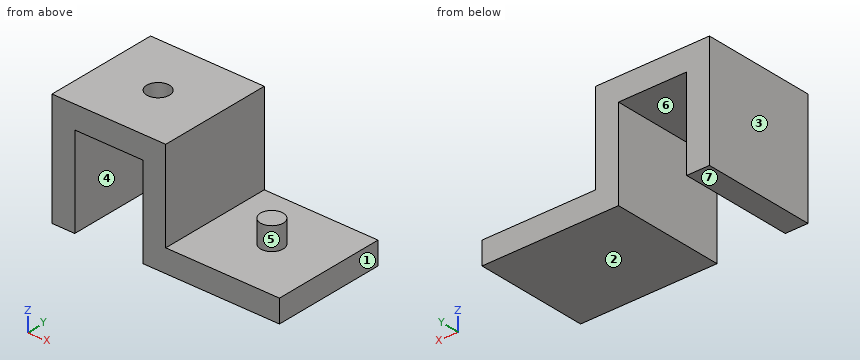
```python
from build123d import *

# Parameters (mm, degrees)
F1_DEPTH = 50
F2_W     = 30
F2_H     = 40
F3_DEPTH = 50.001
F4_R     = 5
F5_DEPTH = 50.001
F6_R     = 5
F7_DEPTH = 10


with BuildPart() as f1:
    # F0 (on Front) → F1 (new body)
    with BuildSketch(Plane.XZ):
        Polygon((0, 50), (0, 0), (100, 0), (100, 10), (50, 10), (50, 50), align=None)
    extrude(amount=F1_DEPTH)

    # F2 (on face) → F3 (cut, through all)
    with BuildSketch(Plane.XZ.offset(50)):
        with Locations((25, 20)):
            Rectangle(F2_W, F2_H)
    extrude(amount=-F3_DEPTH, mode=Mode.SUBTRACT)

    # F4 (on face) → F5 (cut, through all)
    with BuildSketch(Plane.XY.offset(50)):
        with Locations((25, -25)):
            Circle(F4_R)
    extrude(amount=-F5_DEPTH, mode=Mode.SUBTRACT)

    # F6 (on face) → F7 (join)
    with BuildSketch(Plane.XY.offset(10)):
        with Locations((75, -25)):
            Circle(F6_R)
    extrude(amount=F7_DEPTH)


solid = f1.part
```
Here's how the part is built. I have some questions about the finished solid (model axes, mm). Face numbers are marked on the shaded views. A direction names the side the tool comes from. Coordinates: 2 decimals unless noted, no trailing zeros. Write each loop counter-clockwise with the first axis right and the second up, starting at its lowest first coordinate (ties: lowest second). Pieces come first, ordered by that corner, then holes. Notation, with made-up numbers: (-33, 20.5) -> (-28, 20.5) arc R17 ccw to (-28, 26.5) -> close; hole circle Ø8 at (82.25, -11.5). An arc over 180 degrees is marked (long way). Use a Markdown table: item, result. Add a question column.
(1) If we section it at A-A, the plane y = -25: Write out the boundary of the cut face in (x, z), and give its area (3 significant figures).
(2) I'm going to push flat-ended pins straight in: P1, Ø3, axis at x = 76, y = -25, coming from the +Z side; P2, Ø16, axis at x = 25, y = -25, coming from the -Z side; P3, Ø1.5, axis at y = -15, z = 17.5, coming from the +X side. Where does each tip first touch, or does it pass through?
(3) If we section it at D-D, the plane z = 13: Write out the boundary of the cut face in (x, y), and give its area (3 significant figures).
(4) Please list where these lines run through material, in increasing order: line 1 (Y direction, x = 25, z = 45); line 2 (X direction, y = -1.5, z = 25); line 3 (X direction, y = -31, z = 6).
(5) For the marked faces 5, 6 and 7, which set-ups out of +Z, -Z, +X, -X, +Y, -Y let a thin tool reach every point of the face, with its end or its side?
(6) If we section it at B-B, the plane z = 34: Write out the boundary of the cut face in (x, y).
(7) We'd pull the mould along X, two halves only. Please class the marked faces 1, 2, 3 and 4: +X half, -X half, draft (parallel to the pull), parting line (faces both ways), or undercut.
(8) If we section it at C-C, the plane x = 25: Write out the boundary of the cut face in (y, z).
Outcome:
| question | item | result |
|---|---|---|
| 1 | outline | (0, 0) -> (10, 0) -> (10, 40) -> (20, 40) -> (20, 50) -> (0, 50) -> close; (30, 40) -> (40, 40) -> (40, 0) -> (100, 0) -> (100, 10) -> (80, 10) -> (80, 20) -> (70, 20) -> (70, 10) -> (50, 10) -> (50, 50) -> (30, 50) -> close |
| 1 | area | 1,800 mm^2 |
| 2 | P1 | stops at z = 20 |
| 2 | P2 | stops at z = 40 |
| 2 | P3 | stops at x = 50 |
| 3 | outline | (0, -50) -> (10, -50) -> (10, 0) -> (0, 0) -> close; (40, -50) -> (50, -50) -> (50, 0) -> (40, 0) -> close; circle Ø10 at (75, -25) |
| 3 | area | 1,080 mm^2 |
| 4 | line 1 | y = -50 to -30, -20 to 0 |
| 4 | line 2 | x = 0 to 10, 40 to 50 |
| 4 | line 3 | x = 0 to 10, 40 to 100 |
| 5 | face 5 | +Z |
| 5 | face 6 | -Z, +Y, -Y |
| 5 | face 7 | -Z, +X, -X, +Y, -Y |
| 6 | outline | (0, -50) -> (10, -50) -> (10, 0) -> (0, 0) -> close; (40, -50) -> (50, -50) -> (50, 0) -> (40, 0) -> close |
| 7 | face 1 | +X half |
| 7 | face 2 | draft |
| 7 | face 3 | -X half |
| 7 | face 4 | undercut |
| 8 | outline | (-50, 40) -> (-30, 40) -> (-30, 50) -> (-50, 50) -> close; (-20, 40) -> (0, 40) -> (0, 50) -> (-20, 50) -> close |
